from build123d import *

# Parameters (mm, degrees)
SKETCH1_W           = 140
SKETCH1_H           = 30
SKETCH1_R           = 1.9
SKETCH1_W_2         = 60
SKETCH1_H_2         = 6.35
BOSS_EXTRUDE1_DEPTH = 6.35


with BuildPart() as part:
    # Sketch1 → Boss-Extrude1 (new body)
    with BuildSketch(Plane(origin=(0, 0, 0), x_dir=(1, 0, 0), z_dir=(0, 1, 0))):
        with Locations((0, -2.433171599)):
            Rectangle(SKETCH1_W, SKETCH1_H)
        with Locations((38.1, -2.433171599)):
            Circle(SKETCH1_R, mode=Mode.SUBTRACT)
        with Locations((-3.8, -2.433171599)):
            Rectangle(SKETCH1_W_2, SKETCH1_H_2, mode=Mode.SUBTRACT)
    extrude(amount=BOSS_EXTRUDE1_DEPTH)


solid = part.part
Geometry: final body of the model. Coordinates: model frame, mm. A direction names the side the tool comes from. Round coordinates to 2 decimals unless told otherwise and drop trailing zeros. Loops run counter-clockwise (first coordinate to the right, second up) from the corner with the lowest first, then second, coordinate; pieces in that order, holes last.
Q1. Pin query (flat end, axial travel): P1, Ø12, axis at x = -43, z = -8, coming from the -Y side. Return the tip coordinate at first contact, or that it passes through.
Q2. Section C-C on x = 38.1. Return loops of the section in (y, z), plus the area to 3 significant figures.
Q3. Section A-A on x = -23. Return loops of the section in (y, z), plus the area to 3 significant figures.
Q4. Access query for faces 4 (the flat face through (-70, 3, 3)), 5 (the flat face through (-33.8, 3, 2)). Directions: +Z, -Z, +X, -X, +Y, -Y. A direction counts if a zero-diameter tool reaches every point of the face in a straight line with its end or side. Return the directions, or none.
Q5. Material intervals for L1, parallel to Z at x = 38.1, y = 4.5; L2, parallel to Z at x = 9, y = 2; L3, parallel to X at y = 4.25, z = 5, sorted ascending.
Q6. Section B-B on y = 1. Return loops of the section in (x, z), plus the area to 3 significant figures.
Q7. Pull-direction query (Z, two-part tool) for faces 1 (the flat face through (-4, 3, 5.608)), 2 (the flat face through (-1, 0, -1)), 3 (the flat face through (-1, 3, 17.433)); classes: released by +Z, released by -Z, zero draft, split by the parting line, or undercut.
Evaluation:
1. P1: stops at y = 0
2. outline: (0, -12.57) - (6.35, -12.57) - (6.35, 0.53) - (0, 0.53) - close; (0, 4.33) - (6.35, 4.33) - (6.35, 17.43) - (0, 17.43) - close
2. area: 166 mm2
3. outline: (0, -12.57) - (6.35, -12.57) - (6.35, -0.74) - (0, -0.74) - close; (0, 5.61) - (6.35, 5.61) - (6.35, 17.43) - (0, 17.43) - close
3. area: 150 mm2
4. face 4: +Z, -Z, -X, +Y, -Y
4. face 5: +Y, -Y
5. L1: z = -12.57 to 0.53, 4.33 to 17.43
5. L2: z = -12.57 to -0.74, 5.61 to 17.43
5. L3: x = -70 to -33.8, 26.2 to 70
6. outline: (-70, -12.57) - (70, -12.57) - (70, 17.43) - (-70, 17.43) - close; hole (-33.8, -0.74) - (26.2, -0.74) - (26.2, 5.61) - (-33.8, 5.61) - close; hole circle Ø3.8 at (38.1, 2.43)
6. area: 3,810 mm2
7. face 1: undercut
7. face 2: zero draft
7. face 3: released by +Z
